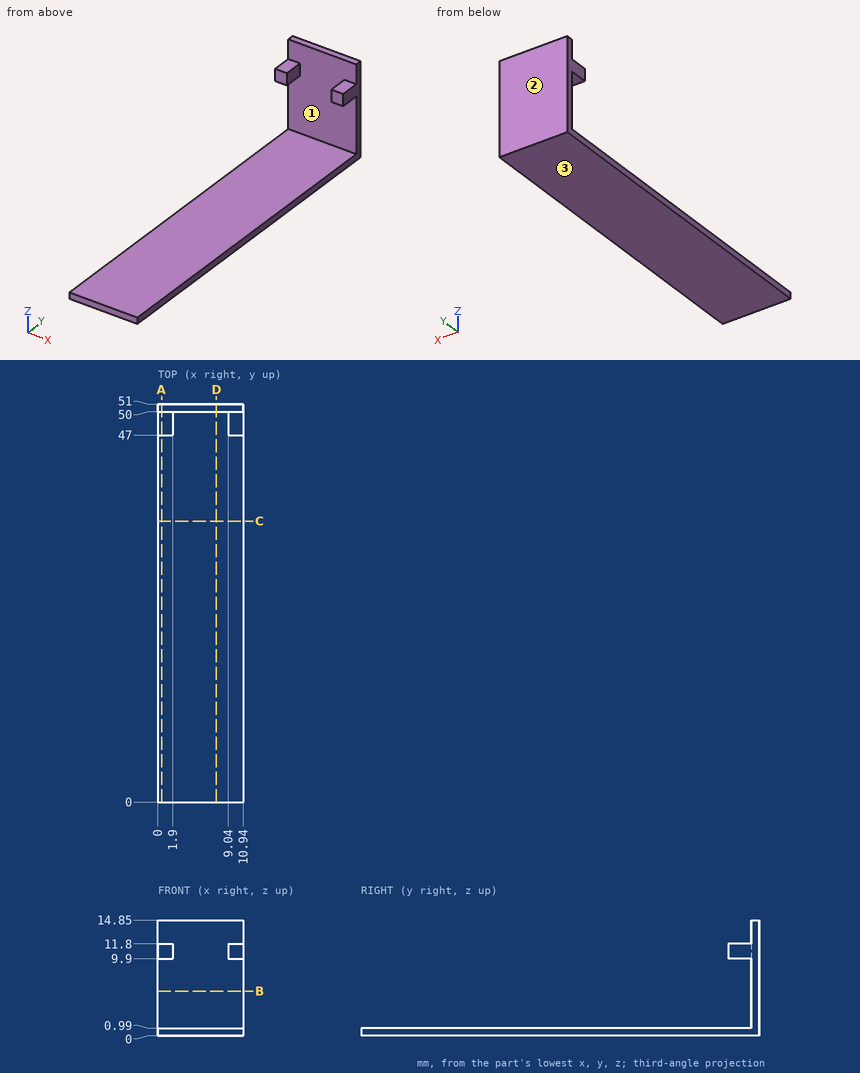
The drawing under review shows one solid part. Ordinate dimensions are in mm from its lowest x, y, z. Round coordinates to 2 decimals unless told otherwise and drop trailing zeros. Write each loop counter-clockwise with the first axis right and the second up, starting at its lowest first coordinate (ties: lowest second). Pieces come first, ordered by that corner, then holes. Notation, with made-up numbers: (15.25, 72.5) -> (70.25, 72.5) arc R6 ccw to (70.25, 76.5) -> close; hole circle Ø1 at (68.5, 69.5). An arc over 180 degrees is marked (long way). One line per question, with ' | ' between items. Start each with the question number.
(1) Add section B-B, the plane z = 5.75. Write out the cut boundary in (x, y).
(2) Insertion check: P1, Ø2, axis at x = 2.5, y = 31.5, coming from the +Z side; P2, Ø1, axis at x = 10, y = 48.5, coming from the +Z side; P3, Ø3.5, axis at x = 7.5, z = 4.5, coming from the -Y side. Each pin has a flat end and moves straight along its axis. Give the tip position at first contact, or say it passes through.
(3) Add section C-C, the plane y = 36. Write out the cut boundary in (x, z).
(4) Mouldability with a two-part tool opening along Z and no side actions: class the marked faces 1, 2 and 3 as released by +Z, released by -Z, zero draft, split by the parting line, or undercut.
(5) For line 1 along Y through (x, z) = (10, 6.75); line 2 along Z through (x, y) = (10.75, 24.5), list the stretches that pass through material, from the lowest coordinate up. Write a range as from..to.
(6) Add section D-D, the plane x = 7.5. Write out the cut boundary in (y, z).
(7) Add section A-A, the plane x = 0.5. Write out the cut boundary in (y, z).
Answer list:
1) outline: (0, 50) -> (10.94, 50) -> (10.94, 51) -> (0, 51) -> close
2) P1: z = 0.99 | P2: z = 11.8 | P3: y = 50
3) outline: (0, 0) -> (10.94, 0) -> (10.94, 0.99) -> (0, 0.99) -> close
4) face 1: undercut | face 2: zero draft | face 3: released by -Z
5) line 1: 50..51 | line 2: 0..0.99
6) outline: (0, 0) -> (51, 0) -> (51, 14.85) -> (50, 14.85) -> (50, 0.99) -> (0, 0.99) -> close
7) outline: (0, 0) -> (51, 0) -> (51, 14.85) -> (50, 14.85) -> (50, 11.8) -> (47, 11.8) -> (47, 9.9) -> (50, 9.9) -> (50, 0.99) -> (0, 0.99) -> close
